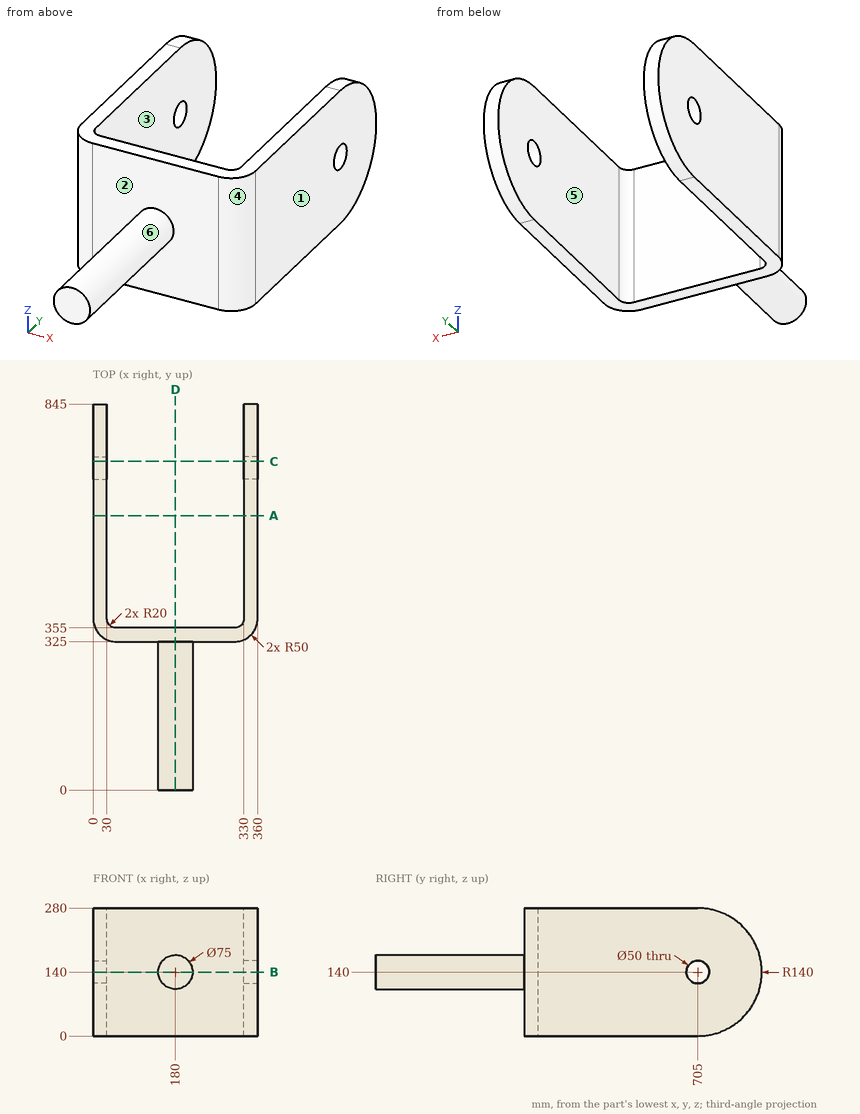
Study the drawing (mm; zero at the part's minimum x, y, z) and answer. A direction names the side the tool comes from. Round coordinates to 2 decimals unless told otherwise and drop trailing zeros. Write each loop counter-clockwise with the first axis right and the second up, starting at its lowest first coordinate (ties: lowest second). Pieces come first, ordered by that corner, then holes. Notation, with made-up numbers: (56.25, -5.5) - (73.25, -5.5) arc R29 ccw to (73.25, 21.5) - close; hole circle Ø5 at (8, 10.5). An arc over 180 degrees is marked (long way). Use CSV: the item, a comma, the result in double quotes.
Q1. Find section C-C, the plane y = 719.5. Write down the section's boundary in (x, z), then the cut area to 3 significant figures.
Values:
outline,"(0, 0.75) - (30, 0.75) - (30, 119.63) - (0, 119.63) - close; (0, 160.37) - (30, 160.37) - (30, 279.25) - (0, 279.25) - close; (330, 0.75) - (360, 0.75) - (360, 119.63) - (330, 119.63) - close; (330, 160.37) - (360, 160.37) - (360, 279.25) - (330, 279.25) - close"
area,"14,300 mm²"
Q2. Each of these flat-tipped pins is pushed along its axis until it touches: pin 1 Ø10 at (y, z) = (357.5, 242) entering from -X; pin 2 Ø4 at (x, z) = (105, 187.5) entering from -Y; pin 3 Ø4 at (x, z) = (50.5, 159.5) entering from +Y. Where does it stop, or does it pass through?
Values:
pin 1,"stops at x = 1.59"
pin 2,"stops at y = 325"
pin 3,"stops at y = 355.06"
Q3. A tool of negligible diameter and unlimited length cuts with its end or side. For the marked faces 4, 5 and 6, from which of +Z, -Z, +X, -X, +Y, -Y can it reach the whole face along a straight path? Write none if from no direction.
Values:
face 4,"+Z, -Z, +X, -Y"
face 5,"+Z, -Z, +Y"
face 6,"-Y"
Q4. Determine the mould class of the marked faces 1, 2 and 3 for opening direction X: +X half, -X half, draft (parallel to the pull), parting line (faces both ways), or undercut.
Values:
face 1,"+X half"
face 2,"draft"
face 3,"undercut"
Q5. Find section A-A, the plane y = 600.5. Write down the section's boundary in (x, z), then the cut area to 3 significant figures.
Values:
outline,"(0, 0) - (30, 0) - (30, 280) - (0, 280) - close; (330, 0) - (360, 0) - (360, 280) - (330, 280) - close"
area,"16,800 mm²"
Q6. Find section D-D, the plane x = 180. Write down the section's boundary in (y, z), then the cut area to 3 significant figures.
Values:
outline,"(0, 102.5) - (325, 102.5) - (325, 0) - (355, 0) - (355, 280) - (325, 280) - (325, 177.5) - (0, 177.5) - close"
area,"32,800 mm²"
Q7. Straight lines are drawn through the part: line 1 along X through (y, z) = (525, 265.5); line 2 along Z through (x, y) = (337.5, 705); line 3 along Y through (x, z) = (99, 180). For each, find the intervals that lie inside material, in ascending order.
Values:
line 1,"x = 0 to 30, 330 to 360"
line 2,"z = 0 to 115, 165 to 280"
line 3,"y = 325 to 355"
Q8. Find section B-B, the plane z = 140. Write down the section's boundary in (x, y), then the cut area to 3 significant figures.
Values:
outline,"(0, 375) arc R50 ccw to (50, 325) - (142.5, 325) - (142.5, 0) - (217.5, 0) - (217.5, 325) - (310, 325) arc R50 ccw to (360, 375) - (360, 680) - (330, 680) - (330, 375) arc R20 cw to (310, 355) - (50, 355) arc R20 cw to (30, 375) - (30, 680) - (0, 680) - close; (0, 730) - (30, 730) - (30, 845) - (0, 845) - close; (330, 730) - (360, 730) - (360, 845) - (330, 845) - close"
area,"60,700 mm²"
